```python
from build123d import *

# Parameters (mm, degrees)
F0_W     = 26.82
F0_H     = 17.02
F1_DEPTH = 0.11
F2_W     = 24.08
F2_H     = 14.28
F3_DEPTH = 0.11
F5_DEPTH = 0.34


with BuildPart() as f1:
    # F0 (on Top) → F1 (new body)
    with BuildSketch(Plane.XY):
        with Locations((1.121439, -2.320423)):
            Rectangle(F0_W, F0_H)
    extrude(amount=F1_DEPTH)

    # F2 (on face) → F3 (join)
    with BuildSketch(Plane.XY.offset(0.11)):
        with Locations((1.121439, -2.320423)):
            Rectangle(F2_W, F2_H)
    extrude(amount=F3_DEPTH)

    # F4 (on face) → F5 (join)
    with BuildSketch(Plane.XY.offset(0.22)):
        with BuildLine():
            Line((3.621439, 0.679577), (-1.378561, 0.679577))
            ThreePointArc((-1.378561, 0.679577), (-1.732114, 0.53313), (-1.878561, 0.179577))
            Line((-1.878561, 0.179577), (-1.878561, -4.820423))
            ThreePointArc((-1.878561, -4.820423), (-1.732114, -5.173977), (-1.378561, -5.320423))
            Line((-1.378561, -5.320423), (3.621439, -5.320423))
            ThreePointArc((3.621439, -5.320423), (3.974992, -5.173977), (4.121439, -4.820423))
            Line((4.121439, -4.820423), (4.121439, 0.179577))
            ThreePointArc((4.121439, 0.179577), (3.974992, 0.53313), (3.621439, 0.679577))
        make_face()
    extrude(amount=F5_DEPTH)


solid = f1.part
```
Model file for the job. Use its own axes, mm. A direction names the side the tool comes from. Coordinates: 2 decimals unless noted, no trailing zeros. Order: outer loops, then holes, each group sorted by start corner. A loop starts at its lowest first (then second) coordinate and runs counter-clockwise, first axis right, second up. Notation, with made-up numbers: (44.5, 62.25) -> (52.5, 62.25) arc R17 cw to (52.5, 74.25) -> close; hole circle Ø4 at (85, 41). An arc over 180 degrees is marked (long way). Return JSON: item names as keys, results as strings.
Item 1: Slice it at B-B (y = -3.5). Write the cut outline in (x, z).
Model answer:
{"outline": "(-12.29, 0) -> (14.53, 0) -> (14.53, 0.11) -> (13.16, 0.11) -> (13.16, 0.22) -> (4.12, 0.22) -> (4.12, 0.56) -> (-1.88, 0.56) -> (-1.88, 0.22) -> (-10.92, 0.22) -> (-10.92, 0.11) -> (-12.29, 0.11) -> close"}
Item 2: Wall check: line 1 along Z through (x, y) = (-7.5, -1.75); line 2 along X through (y, z) = (-3, 0.25); line 3 along X through (y, z) = (-7, 0.15). Give the ranges that are in metal, low to high. Write a range as from..to.
Model answer:
{"line 1": "z = 0..0.22", "line 2": "x = -1.88..4.12", "line 3": "x = -10.92..13.16"}
Item 3: Pin check, flat tip, straight feed: P1, Ø5, axis at x = 7, y = 1, coming from the +Z side. Stop position of the tip, or through.
Model answer:
{"P1": "stops at z = 0.22"}
Item 4: 3-axis set-ups, long thin cutter, end or side, ignore diameter. For faces 1 (the face through (1, -2, 0)), 2 (the face through (1, 1, 0.22)): which of +Z, -Z, +X, -X, +Y, -Y reach the whole face in a straight line?
Model answer:
{"face 1": "-Z, +X, -X, +Y, -Y", "face 2": "+Z"}
Item 5: Slice it at D-D (y = -6.5). Write the cut outline in (x, z), then the cut area to 3 significant figures.
Model answer:
{"outline": "(-12.29, 0) -> (14.53, 0) -> (14.53, 0.11) -> (13.16, 0.11) -> (13.16, 0.22) -> (-10.92, 0.22) -> (-10.92, 0.11) -> (-12.29, 0.11) -> close", "area": "5.60 mm²"}
Item 6: Slice it at C-C (z = 0.45). Write the cut outline in (x, y).
Model answer:
{"outline": "(-1.88, -4.82) arc R0.5 ccw to (-1.38, -5.32) -> (3.62, -5.32) arc R0.5 ccw to (4.12, -4.82) -> (4.12, 0.18) arc R0.5 ccw to (3.62, 0.68) -> (-1.38, 0.68) arc R0.5 ccw to (-1.88, 0.18) -> close"}
Item 7: Slice it at A-A (x = 2.25). Write the cut outline in (y, z).
Model answer:
{"outline": "(-10.83, 0) -> (6.19, 0) -> (6.19, 0.11) -> (4.82, 0.11) -> (4.82, 0.22) -> (0.68, 0.22) -> (0.68, 0.56) -> (-5.32, 0.56) -> (-5.32, 0.22) -> (-9.46, 0.22) -> (-9.46, 0.11) -> (-10.83, 0.11) -> close"}
